from build123d import *

# Parameters (mm, degrees)
CROQUIS1_R              = 2.1
SALIENTE_EXTRUIR1_DEPTH = 4
CROQUIS1_6_R            = 2.1
SALIENTE_EXTRUIR3_DEPTH = 12.2
REDONDEO1_R             = 10
REDONDEO2_R             = 1


with BuildPart() as part:
    # Croquis1 → Saliente-Extruir1 (new body)
    with BuildSketch(Plane.XY):
        with BuildLine():
            ThreePointArc((10, 54), (0, 64), (-10, 54))
            Line((-10, 54), (-10, -54))
            ThreePointArc((-10, -54), (0, -64), (10, -54))
            Line((10, -54), (10, 54))
        make_face()
        with Locations((0, 54)):
            Circle(CROQUIS1_R, mode=Mode.SUBTRACT)
        with BuildLine():
            Line((6, 38), (6, 22))
            Line((6, 22), (-6, 34))
            Line((-6, 34), (-6, 38))
            ThreePointArc((-6, 38), (0, 44), (6, 38))
        make_face(mode=Mode.SUBTRACT)
        Polygon((6, 16), (6, -16), (-6, -4), (-6, 4), align=None, mode=Mode.SUBTRACT)
        with BuildLine():
            Line((6, -22), (6, -38))
            ThreePointArc((6, -38), (0, -44), (-6, -38))
            Line((-6, -38), (-6, -34))
            Line((-6, -34), (6, -22))
        make_face(mode=Mode.SUBTRACT)
        Polygon((-6, -31), (-6, -7), (6, -19), align=None, mode=Mode.SUBTRACT)
        Polygon((-6, 7), (-6, 31), (6, 19), align=None, mode=Mode.SUBTRACT)
        with Locations((0, -54)):
            Circle(CROQUIS1_R, mode=Mode.SUBTRACT)
    extrude(amount=SALIENTE_EXTRUIR1_DEPTH)

    # Croquis1<6> → Saliente-Extruir3 (add)
    with BuildSketch(Plane.XY):
        with BuildLine():
            Line((10, 47.95), (10, 54))
            ThreePointArc((10, 54), (0, 64), (-10, 54))
            Line((-10, 54), (-10, 47.95))
            Line((-10, 47.95), (10, 47.95))
        make_face()
        with Locations((0, 54)):
            Circle(CROQUIS1_6_R, mode=Mode.SUBTRACT)
    extrude(amount=SALIENTE_EXTRUIR3_DEPTH)

    # Redondeo1
    # the kernel refuses this fillet: 10 mm, written as the material it adds along each edge
    with BuildSketch(Plane(origin=(10, 47.95, 4), x_dir=(0, 0, 1), z_dir=(-1, 0, 0))) as redondeo1_piece_1_section:
        with BuildLine():
            CenterArc((10, -9.836666102), REDONDEO1_R, 100.369759805, 79.630240195)
            Line((0, -9.836666102), (-0.2, -9.836666102))
            Line((-0.2, -9.836666102), (-0.2, 0))
            Line((-0.2, 0), (0, 0.2))
            ThreePointArc((0, 0.2), (4.1, 0.2), (8.164, 0.196733322))
            Line((8.164, 0.196733322), (8.2, 0))
        make_face()
    redondeo1_piece_1 = extrude(amount=20, mode=Mode.PRIVATE)
    redondeo1_piece_1 = redondeo1_piece_1 - Plane(origin=(0, 38, 6.176378177), x_dir=(-1, 0, 0), z_dir=(0, 0, -1)) * Cylinder(6, 80, mode=Mode.PRIVATE)
    add(redondeo1_piece_1)

    # Redondeo2
    redondeo2_edges = [part.edges().sort_by_distance(p)[0] for p in [
        (6, 22, 2),
        (-6, 34, 2),
        (6, -22, 2),
        (-6, -34, 2),
        (-6, -31, 2),
        (6, -19, 2),
        (-6, -7, 2),
        (-6, -4, 2),
        (6, -16, 2),
        (6, 16, 2),
        (-6, 4, 2),
        (-6, 7, 2),
        (6, 19, 2),
        (-6, 31, 2),
    ]]
    fillet(redondeo2_edges, radius=REDONDEO2_R)


solid = part.part
The model under review builds one solid part; all positions refer to its coordinate system, in mm. A direction names the side the tool comes from. Round coordinates to 2 decimals unless told otherwise and drop trailing zeros. Order: outer loops, then holes, each group sorted by start corner. A loop starts at its lowest first (then second) coordinate and runs counter-clockwise, first axis right, second up. Notation, with made-up numbers: (-12, 65) - (1, 65) arc R16 ccw to (1, 84) - close; hole circle Ø10 at (71.25, 69). An arc over 180 degrees is marked (long way). Use one line per item in the form item = value.
Q1. Add section B-B on y = -26. Give the boundary of the cut face in (x, z).
Response values:
outline = (-10, 0) - (-6, 0) - (-6, 4) - (-10, 4) - close; (-1, 0) - (2, 0) - (2, 4) - (-1, 4) - close; (6, 0) - (10, 0) - (10, 4) - (6, 4) - close
Q2. Mouldability with a two-part tool opening along X and no side actions: class faces 3 (the flat face through (10, 13, 3)), 4 (the flat face through (-6, -19, 2)), 5 (the flat face through (-10, 13, 3)), 6 (the cylindrical face through (0, 64, 6)) as pulls with the +X half, pulls with the -X half, needs draft (parallel to the pull), parting line crosses it, or undercut.
Response values:
face_3 = pulls with the +X half
face_4 = undercut
face_5 = pulls with the -X half
face_6 = parting line crosses it
Q3. Add section C-C on y = 36.5. Give the boundary of the cut face in (x, z).
Response values:
outline = (-10, 0) - (-6, 0) - (-6, 4) - (-10, 4) - close; (6, 0) - (10, 0) - (10, 4) - (6, 4) - close
Q4. Clearance check with flat-ended pins moving along their axes: P1, Ø3, axis at x = -1.5, z = 6, coming from the +Y side; P2, Ø4, axis at x = 0.5, z = 10.5, coming from the -Y side (3 decimals). State where each tip first meets the part, or that it passes through.
Response values:
P1 = 64
P2 = 46.465
Q5. To check wall thickness, follow line 1 (X direction, y = -28, z = 0.75); line 2 (Z direction, x = -7.5, y = 13.5); line 3 (X direction, y = 52.5, z = 3.25). State the ranges of each line that lie inside material, in increasing order.
Response values:
line_1 = -10 to -6, -3 to 0, 6 to 10
line_2 = 0 to 4
line_3 = -10 to -1.47, 1.47 to 10
Q6. Add section D-D on z = 10.75. Give the boundary of the cut face in (x, y), then the cut area to 3 significant figures.
Response values:
outline = (-10, 47.57) - (10, 47.57) - (10, 54) arc R10 ccw to (-10, 54) - close; hole circle Ø4.2 at (0, 54)
area = 272 mm^2
Q7. Tool access review of faces 1 (the cylindrical face through (0, 44, 2)), 2 (the cylindrical face through (0, -64, 2)): name each direction out of +Z, -Z, +X, -X, +Y, -Y from which nothing blocks a thin tool from reaching the whole face with its end or side.
Response values:
face_1 = +Z, -Z
face_2 = +Z, -Z, -Y
Q8. Add section A-A on x = 0. Give the number of separate pieces and of enclosed holes in the cut face, then the cut area to 3 significant figures.
Response values:
separate_pieces = 8
enclosed_holes = 0
area = 288 mm^2
